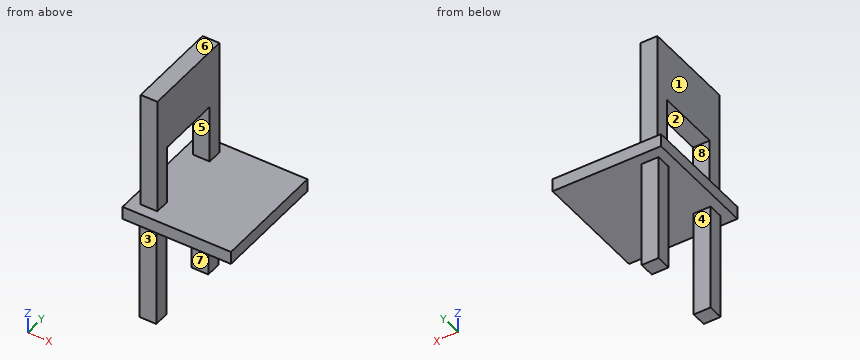
from build123d import *

# Parameters (mm, degrees)
F0_W      = 106.4638644457
F0_H      = 103.2169535756
F1_DEPTH  = 12.7
F2_W      = 16.3826718926
F2_H      = 14.1792520881
F3_DEPTH  = 115.4824048281
F4_W      = 16.3826718926
F4_H      = 57.741202414
F5_DEPTH  = 25.4
F7_DEPTH  = 12.7457336903
F8_W      = 16.5637210011
F8_H      = 14.8448646069
F9_DEPTH  = 106.4620614052
F10_R     = 29.9454441035
F11_DEPTH = 25.4


with BuildPart() as f1:
    # F0 (on Top) → F1 (new body)
    with BuildSketch(Plane.XY):
        with Locations((3.0183121562, -5.1516257226)):
            Rectangle(F0_W, F0_H)
    extrude(amount=F1_DEPTH)

    # F2 (on face) → F3 (join)
    with BuildSketch(Plane.XY.offset(12.7)):
        with Locations((-31.3676968217, -38.8624928892)):
            Rectangle(F2_W, F2_H)
    extrude(amount=F3_DEPTH)

    # F4 (on face) → F5 (join)
    with BuildSketch(Plane(origin=(0, -31.7728668451, 0), x_dir=(-1, 0, 0), z_dir=(0, 1, 0))):
        with Locations((31.3676968217, 99.3118036211)):
            Rectangle(F4_W, F4_H)
    extrude(amount=F5_DEPTH)

    # F6: F1 across plane


with BuildPart() as f1_1:
    add(f1.part)
    add(f1.part.mirror(Plane.XZ))

    # F7 (add, through all): a face of the model
    f7_faces = [f1_1.faces().sort_by_distance(p)[0] for p in [
        (-31.3676968217, -6.3728668451, 99.3118036211),
    ]]
    extrude(f7_faces, amount=F7_DEPTH)

    # F8 (on face) → F9 (join)
    with BuildSketch(Plane(origin=(0, 0, 0), x_dir=(1, 0, 0), z_dir=(0, 0, -1))):
        with Locations((-32.4887447059, 38.6229231954)):
            Rectangle(F8_W, F8_H)
    extrude(amount=F9_DEPTH)

    # F13: F1 across plane


with BuildPart() as f11:
    # F10 (on Top) → F11 (new body)
    with BuildSketch(Plane.XY):
        with Locations((108.9618206024, 20.2722847462)):
            Circle(F10_R)
    extrude(amount=F11_DEPTH)


with BuildPart() as f1_2:
    add(f1_1.part)
    add(f1_1.part.mirror(Plane.XZ))


solid = f1_2.part
Build history of the part. All positions in model axes, mm. Face numbers are marked on the shaded views. A direction names the side the tool comes from. Give positions to 0.01 mm unless a question says otherwise; leave off trailing zeros. Write each loop counter-clockwise with the first axis right and the second up, starting at its lowest first coordinate (ties: lowest second). Pieces come first, ordered by that corner, then holes. Notation, with made-up numbers: (65.25, 66.5) - (107.25, 66.5) arc R20 ccw to (107.25, 105.5) - close; hole circle Ø6 at (42.5, -35.5). An arc over 180 degrees is marked (long way). Use one line per item in the form item = value. Start each with the question number.
1. Band-saw the part on D-D on y = -35. Write the cut outline in (x, z), plus the area to 3 significant figures.
2. Drop flat-ended pins along their axis: pin 1 Ø6 at (x, y) = (9.5, -4) entering from -Z; pin 2 Ø13.5 at (x, z) = (-30, -37.5) entering from +Y; pin 3 Ø7.5 at (y, z) = (36, -65) entering from +X. Give the stop position or say it passes through.
3. Two-plate mould, pull along Z, no slides. Class the marked faces 5, 6, 7 and 8: released by +Z, released by -Z, zero draft, split by the parting line, or undercut.
4. Band-saw the part on A-A on z = 33. Write the cut outline in (x, y), plus the area to 3 significant figures.
5. Probe line 1 (Y direction, x = -29, z = -37.5); line 2 (Z direction, x = 10, y = -15); line 3 (X direction, y = -31.5, z = -2.5). List the from-to ranges inside material, lowest first. Write a range as [from, to].
6. 3-axis set-ups, long thin cutter, end or side, ignore diameter. For the marked faces 1, 2, 3 and 4: which of +Z, -Z, +X, -X, +Y, -Y reach the whole face in a straight line?
7. Band-saw the part on C-C on y = 19. Write the cut outline in (x, z).
8. Band-saw the part on B-B on x = -36. Write the cut outline in (y, z), plus the area to 3 significant figures.
Conclusion:
q1.outline = (-50.21, 0) - (-40.77, 0) - (-40.77, -106.46) - (-24.21, -106.46) - (-24.21, 0) - (56.25, 0) - (56.25, 12.7) - (-23.18, 12.7) - (-23.18, 128.18) - (-39.56, 128.18) - (-39.56, 12.7) - (-50.21, 12.7) - close
q1.area = 5,010 mm²
q2.pin_1 = 0
q2.pin_2 = 46.05
q2.pin_3 = -24.21
q3.face_5 = undercut
q3.face_6 = released by +Z
q3.face_7 = zero draft
q3.face_8 = undercut
q4.outline = (-39.56, -45.95) - (-23.18, -45.95) - (-23.18, -31.77) - (-39.56, -31.77) - close; (-39.56, 31.77) - (-23.18, 31.77) - (-23.18, 45.95) - (-39.56, 45.95) - close
q4.area = 465 mm²
q5.line_1 = [-46.05, -31.2], [31.2, 46.05]
q5.line_2 = [0, 12.7]
q5.line_3 = [-40.77, -24.21]
q6.face_1 = +Z, -X, +Y, -Y
q6.face_2 = +X, -X
q6.face_3 = -Z, +X, -X, -Y
q6.face_4 = -Z, +X, -X
q7.outline = (-50.21, 0) - (56.25, 0) - (56.25, 12.7) - (-50.21, 12.7) - close; (-39.56, 70.44) - (-23.18, 70.44) - (-23.18, 128.18) - (-39.56, 128.18) - close
q8.outline = (-56.76, 0) - (-46.05, 0) - (-46.05, -106.46) - (-31.2, -106.46) - (-31.2, 0) - (31.2, 0) - (31.2, -106.46) - (46.05, -106.46) - (46.05, 0) - (56.76, 0) - (56.76, 12.7) - (45.95, 12.7) - (45.95, 128.18) - (-45.95, 128.18) - (-45.95, 12.7) - (-56.76, 12.7) - close; hole (-31.77, 12.7) - (31.77, 12.7) - (31.77, 70.44) - (-31.77, 70.44) - close
q8.area = 11,500 mm²
